Model file for the job. Use its own axes, mm. A direction names the side the tool comes from. Coordinates: 2 decimals unless noted, no trailing zeros.
from build123d import *

# Parameters (mm, degrees)
SKETCH2_W           = 50
SKETCH2_H           = 9.4
BOSS_EXTRUDE1_DEPTH = 3
BOSS_EXTRUDE2_DEPTH = 3
CUT_EXTRUDE1_REACH  = 145.812
SKETCH6_R           = 1.5
SKETCH7_W           = 33
SKETCH7_H           = 25
CUT_EXTRUDE2_DEPTH  = 18.5
CHAMFER1_SIZE       = 3
CUT_EXTRUDE4_REACH  = 145.812
CHAMFER2_SIZE       = 3
CHAMFER3_SIZE       = 3
CUT_EXTRUDE5_REACH  = 145.812
SKETCH9_R           = 1.475
CUT_EXTRUDE6_REACH  = 146.305
CHAMFER4_SIZE       = 8


with BuildPart() as part:
    # Sketch2 → Boss-Extrude1 (new body)
    with BuildSketch(Plane(origin=(0, 0, 0), x_dir=(1, 0, 0), z_dir=(0, 1, 0))):
        Polygon((113, 0), (120, 0), (120, 69), (0, 69), (0, 0), (83, 0), (83, 28), (113, 28), align=None)
        with Locations((80, 57.7)):
            Rectangle(SKETCH2_W, SKETCH2_H, mode=Mode.SUBTRACT)
    extrude(amount=BOSS_EXTRUDE1_DEPTH)

    # Sketch4 → Loft1 section 0
    with BuildSketch(Plane(origin=(0, 39, 0), x_dir=(1, 0, 0), z_dir=(0, 1, 0))):
        with BuildLine():
            Line((11.5, 8), (8, 8))
            Line((8, 8), (8, 64))
            Line((8, 64), (112, 64))
            Line((112, 64), (112, 8))
            Line((112, 8), (108.5, 8))
            Line((108.5, 8), (108.5, 60.5))
            Line((108.5, 60.5), (11.5, 60.5))
            Line((11.5, 60.5), (11.5, 8))
        make_face()
    # Sketch3 → Loft1 section 1
    with BuildSketch(Plane(origin=(0, 3, 0), x_dir=(1, 0, 0), z_dir=(0, 1, 0))):
        with BuildLine():
            Line((3.5, 0), (3.5, 65.5))
            Line((3.5, 65.5), (116.5, 65.5))
            Line((116.5, 65.5), (116.5, 0))
            Line((116.5, 0), (120, 0))
            Line((120, 0), (120, 69))
            Line((120, 69), (0, 69))
            Line((0, 69), (0, 0))
            Line((0, 0), (3.5, 0))
        make_face()
    loft()

    # Sketch5 → Boss-Extrude2 (add)
    with BuildSketch(Plane(origin=(0, 39, 0), x_dir=(1, 0, 0), z_dir=(0, 1, 0))):
        with BuildLine():
            Line((8, 64), (18, 64))
            Line((18, 64), (18, 60))
            ThreePointArc((18, 60), (16.242640687, 55.757359313), (12, 54))
            Line((12, 54), (8, 54))
            Line((8, 54), (8, 64))
        make_face()
        with BuildLine():
            Line((112, 64), (102, 64))
            Line((102, 64), (102, 60))
            ThreePointArc((102, 60), (103.757359313, 55.757359313), (108, 54))
            Line((108, 54), (112, 54))
            Line((112, 54), (112, 64))
        make_face()
    extrude(amount=-BOSS_EXTRUDE2_DEPTH)

    # Sketch6 → Cut-Extrude1 (cut, up to next)
    with BuildSketch(Plane(origin=(0, 39, 0), x_dir=(1, 0, 0), z_dir=(0, 1, 0)), mode=Mode.PRIVATE) as cut_extrude1_sk1:
        with Locations(Location((13.5, 58.5, 0), (0, 0, 270))):
            Circle(SKETCH6_R)
    cut_extrude1_tool1 = extrude(cut_extrude1_sk1.sketch, amount=-CUT_EXTRUDE1_REACH, mode=Mode.PRIVATE) & part.part
    # Sketch6 → Cut-Extrude1 (cut, up to next)
    with BuildSketch(Plane(origin=(0, 39, 0), x_dir=(1, 0, 0), z_dir=(0, 1, 0)), mode=Mode.PRIVATE) as cut_extrude1_sk2:
        with Locations(Location((106.5, 58.5, 0), (0, 0, 270))):
            Circle(SKETCH6_R)
    cut_extrude1_tool2 = extrude(cut_extrude1_sk2.sketch, amount=-CUT_EXTRUDE1_REACH, mode=Mode.PRIVATE) & part.part
    add(cut_extrude1_tool1.solids().sort_by_distance((13.5, 39, -58.5))[0], mode=Mode.SUBTRACT)
    add(cut_extrude1_tool2.solids().sort_by_distance((106.5, 39, -58.5))[0], mode=Mode.SUBTRACT)

    # Sketch7 → Cut-Extrude2 (cut)
    with BuildSketch(Plane.XZ):
        with Locations((10.5, -41.5)):
            Rectangle(SKETCH7_W, SKETCH7_H)
    extrude(amount=-CUT_EXTRUDE2_DEPTH, mode=Mode.SUBTRACT)

    # Chamfer1
    chamfer1_edges = [part.edges().sort_by_distance(p)[0] for p in [
        (55, 0, -57.7),
        (80, 0, -62.4),
        (105, 0, -57.7),
        (80, 0, -53),
    ]]
    chamfer(chamfer1_edges, length=CHAMFER1_SIZE - 0.0001)  # a hair under: the kernel refuses the full size

    # Cut-Extrude4: up to this plane
    cut_extrude4_end = Plane(origin=(0, 8.981831945, -64.669190008), z_dir=(0, -0.1375683712746883, 0.9904922731777515))
    # Sketch8 → Cut-Extrude4 (cut, up to the surface)
    with BuildSketch(Plane(origin=(0, 0, -69), x_dir=(-1, 0, 0), z_dir=(0, 0, -1)), mode=Mode.PRIVATE) as cut_extrude4_sk1:
        Polygon((-27, 3), (-39, 3), (-39, 17.01), (-33.01, 23), (-32.99, 23), (-27, 17.01), align=None)
    cut_extrude4_tool1 = split(extrude(cut_extrude4_sk1.sketch, amount=-CUT_EXTRUDE4_REACH, mode=Mode.PRIVATE), bisect_by=cut_extrude4_end, keep=Keep.BOTH, mode=Mode.PRIVATE)
    add(cut_extrude4_tool1.solids().sort_by_distance((33, 11.593178, -69))[0], mode=Mode.SUBTRACT)

    # Chamfer2
    chamfer2_edges = [part.edges().sort_by_distance(p)[0] for p in [
        (83, 0, -14),
        (113, 0, -14),
        (98, 0, -28),
    ]]
    chamfer(chamfer2_edges, length=CHAMFER2_SIZE - 0.0001)  # a hair under: the kernel refuses the full size

    # Chamfer3
    chamfer3_edges = [part.edges().sort_by_distance(p)[0] for p in [
        (13.5, 0, -54),
        (27, 0, -41.5),
        (13.5, 0, -29),
    ]]
    chamfer(chamfer3_edges, length=CHAMFER3_SIZE - 0.0001)  # a hair under: the kernel refuses the full size

    # Sketch9 → Cut-Extrude5 (cut, up to next)
    with BuildSketch(Plane.XZ, mode=Mode.PRIVATE) as cut_extrude5_sk1:
        with Locations(Location((89.5, -35.6, 0), (0, 0, 270))):
            Circle(SKETCH9_R)
    cut_extrude5_tool1 = extrude(cut_extrude5_sk1.sketch, amount=-CUT_EXTRUDE5_REACH, mode=Mode.PRIVATE) & part.part
    # Sketch9 → Cut-Extrude5 (cut, up to next)
    with BuildSketch(Plane.XZ, mode=Mode.PRIVATE) as cut_extrude5_sk2:
        with Locations(Location((74.5, -35.6, 0), (0, 0, 270))):
            Circle(SKETCH9_R)
    cut_extrude5_tool2 = extrude(cut_extrude5_sk2.sketch, amount=-CUT_EXTRUDE5_REACH, mode=Mode.PRIVATE) & part.part
    add(cut_extrude5_tool1.solids().sort_by_distance((89.5, 0, -35.6))[0], mode=Mode.SUBTRACT)
    add(cut_extrude5_tool2.solids().sort_by_distance((74.5, 0, -35.6))[0], mode=Mode.SUBTRACT)

    # Sketch10 → Cut-Extrude6 (cut, up to next)
    with BuildSketch(Plane(origin=(-0.635294118, 0.141176471, 0), x_dir=(0, 0, 1), z_dir=(-0.9761870601839528, 0.21693045781865627, 0)), mode=Mode.PRIVATE) as cut_extrude6_sk1:
        Polygon((-0.780111958, 20), (-18.610201871, 20), (-18.610201871, 30), (-7.717228125, 40.892973746), align=None)
    cut_extrude6_tool1 = extrude(cut_extrude6_sk1.sketch, amount=-CUT_EXTRUDE6_REACH, mode=Mode.PRIVATE) & part.part
    add(cut_extrude6_tool1.solids().sort_by_distance((5.377692, 27.199615, -10.380545))[0], mode=Mode.SUBTRACT)

    # Chamfer4
    chamfer4_edges = [part.edges().sort_by_distance(p)[0] for p in [
        (5.194444444, 18.5, -29),
        (5.194444444, 18.5, -54),
    ]]
    chamfer(chamfer4_edges, length=CHAMFER4_SIZE)


solid = part.part
Q1. Drill centre lines: line 1 (X direction, y = 1, z = -35); line 2 (X direction, y = 1.65, z = -35.6) (3 decimals); line 3 (Z direction, x = 89, y = 1). Where is each one in solid material? Low to high.
Answers:
line 1: x = 29 to 73.15, 75.85 to 88.15, 90.85 to 120
line 2: x = 28.35 to 73.025, 75.975 to 88.025, 90.975 to 120
line 3: z = -69 to -64.4, -51 to -36.99, -34.21 to -30
Q2. Flat gauge pins, fed straight in: P1, Ø4, axis at x = 17.5, y = 8.5, coming from the -Z side; P2, Ø5, axis at y = 30, z = -40.5, coming from the -X side; P3, Ø3, axis at x = 7.5, y = 25, coming from the +Z side; P4, Ø5, axis at x = 13.5, z = -58.5, coming from the +Y side. Where does each tip first touch, or does it go through?
Answers:
P1: stops at z = -68.51
P2: stops at x = 5.44
P3: stops at z = -18.61
P4: stops at y = 39
Q3. Slice it at A-A (x = 89.5). Count the separate pieces of the cut face and the enclosed holes in it, and give its area (3 significant figures).
Answers:
separate pieces: 3
enclosed holes: 0
area: 198 mm2
Q4. Which spindle directions (+Z, -Z, +X, -X, +Y, -Y) get a long thin tool onto all of the face, cutting with end or side? Do faces 1 (the flat face through (114, 2, -16)), 2 (the cylindrical face through (103.711, 37.521, -55.804)), 3 (the flat face through (5, 18.5, -41)). Say none if no direction does.
Answers:
face 1: +Z, -Y
face 2: +Z, +Y
face 3: -X, -Y
Q5. Mould opens along Y. For faces 4 (the flat face through (120, 1, -34)), 5 (the flat face through (54, 2, -58)), 6 (the flat face through (6, 24, -18.61)) say: +Y half, -Y half, draft (parallel to the pull), parting line (faces both ways), or undercut.
Answers:
face 4: draft
face 5: -Y half
face 6: undercut
